```python
from build123d import *

# Parameters (mm, degrees)
BOSS_EXTRUDE1_DEPTH      = 1.5
SKETCH2_W                = 14
SKETCH2_H                = 32
BOSS_EXTRUDE2_DEPTH      = 16
BOSS_EXTRUDE3_DEPTH      = 3
BOSS_EXTRUDE3_DEPTH_BACK = 0.001
SKETCH3_W                = 15.664729633
SKETCH3_H                = 27
SKETCH3_R                = 1.75
SKETCH5_R                = 2.5
BOSS_EXTRUDE4_DEPTH      = 4
BOSS_EXTRUDE4_TAPER      = 15
CUT_EXTRUDE1_DEPTH       = 10
SKETCH7_W                = 71.065748979
SKETCH7_H                = 70.277880365
CUT_EXTRUDE2_DEPTH       = 30


with BuildPart() as part:
    # Sketch1 → Boss-Extrude1 (new body)
    with BuildSketch(Plane.YZ):
        Polygon((-13.5, 8), (-13.5, -8), (13.5, -8), (13.5, 8), (5, 8), (5, 58), (-5, 58), (-5, 8), align=None)
    extrude(amount=-BOSS_EXTRUDE1_DEPTH)



with BuildPart() as body_2:
    # Sketch2 → Boss-Extrude2 (new body)
    with BuildSketch(Plane.YZ):
        with Locations((0, -24)):
            Rectangle(SKETCH2_W, SKETCH2_H)
    extrude(amount=BOSS_EXTRUDE2_DEPTH)


with BuildPart() as part_1:
    add(part.part)

    add(body_2.part)  # Boss-Extrude3 merges body 2
    # Sketch3 → Boss-Extrude3 (add, two sides: drawn at the far end of the back side and taken through both)
    with BuildSketch(Plane.XY.offset(-8).offset(-BOSS_EXTRUDE3_DEPTH_BACK)):
        with Locations((6.299899253, 0)):
            Rectangle(SKETCH3_W, SKETCH3_H)
        with Locations((9.132264069, 9)):
            Circle(SKETCH3_R, mode=Mode.SUBTRACT)
        with Locations((9.132264069, -9)):
            Circle(SKETCH3_R, mode=Mode.SUBTRACT)
    extrude(amount=BOSS_EXTRUDE3_DEPTH + BOSS_EXTRUDE3_DEPTH_BACK)

    # Sketch5 → Boss-Extrude4 (add)
    with BuildSketch(Plane(origin=(0, 0, -40), x_dir=(1, 0, 0), z_dir=(0, 0, -1))):
        with Locations((9, 0)):
            Circle(SKETCH5_R)
    extrude(amount=BOSS_EXTRUDE4_DEPTH, taper=BOSS_EXTRUDE4_TAPER)

    # Sketch6 → Cut-Extrude1 (cut)
    with BuildSketch(Plane.YZ):
        with BuildLine():
            Line((0.555279177, 48), (0.555279177, 18))
            ThreePointArc((0.555279177, 18), (-1.194720823, 16.25), (-2.944720823, 18))
            Line((-2.944720823, 18), (-2.944720823, 48))
            ThreePointArc((-2.944720823, 48), (-1.194720823, 49.75), (0.555279177, 48))
        make_face()
    extrude(amount=-CUT_EXTRUDE1_DEPTH, mode=Mode.SUBTRACT)

    # Sketch7 → Cut-Extrude2 (cut)
    with BuildSketch(Plane.YZ.offset(14.132264069)):
        with Locations((0.078786861, 30.138940183)):
            Rectangle(SKETCH7_W, SKETCH7_H)
    extrude(amount=-CUT_EXTRUDE2_DEPTH, mode=Mode.SUBTRACT)


solid = part_1.part
```
Input: part model. Units: mm. Frame: model coordinates. A direction names the side the tool comes from. Give positions to 0.01 mm unless a question says otherwise; leave off trailing zeros. Loops run counter-clockwise (first coordinate to the right, second up) from the corner with the lowest first, then second, coordinate; pieces in that order, holes last.
1) Line query: L1, parallel to Z at x = 3.5, y = 9.25; L2, parallel to Y at x = 14, z = -23.5; L3, parallel to X at y = 0.5, z = -15.5. Output: solid intervals per line, ascending.
A:
L1: z = -8 to -5
L2: y = -7 to 7
L3: x = 0 to 16
2) Section query B-B on x = 2.5. Return the cut outline in (y, z).
A:
outline: (-13.5, -8) - (-7, -8) - (-7, -40) - (7, -40) - (7, -8) - (13.5, -8) - (13.5, -5) - (-13.5, -5) - close
3) Section query D-D on z = -34.5. Return the cut outline in (x, y), and give its area (3 significant figures).
A:
outline: (0, -7) - (16, -7) - (16, 7) - (0, 7) - close
area: 224 mm2
4) Section query A-A on y = 9. Return the cut outline in (x, z).
A:
outline: (-1.53, -8) - (7.38, -8) - (7.38, -5) - (-1.53, -5) - close; (10.88, -8) - (14.13, -8) - (14.13, -5) - (10.88, -5) - close
5) Mould query, pull axis X, two halves, no side actions, for faces 5 (the flat face through (0, 0, -24)), 6 (the cylindrical face through (8.904, 10.735, -6.522)), 7 (the flat face through (6, 0, -40)). Classes: released by +X, released by -X, zero draft, split by the parting line, or undercut.
A:
face 5: released by -X
face 6: undercut
face 7: zero draft
6) Section query C-C on x = 9. Return the cut outline in (y, z) (3 decimals).
A:
outline: (-13.5, -8.001) - (-10.745, -8.001) - (-10.745, -5) - (-13.5, -5) - close; (-7.255, -8.001) - (-7, -8.001) - (-7, -40) - (-2.5, -40) - (-1.428, -44) - (1.428, -44) - (2.5, -40) - (7, -40) - (7, -8.001) - (7.255, -8.001) - (7.255, -5) - (-7.255, -5) - close; (10.745, -8.001) - (13.5, -8.001) - (13.5, -5) - (10.745, -5) - close
7) Contact query for flat-ended pins moving along their axis: pin 1 (0.9 mm diameter, centred on x = 15, y = -0.5, fed in from +Z); pin 2 (5 mm diameter, centred on x = 8, z = -29.5, fed in from -Y); pin 3 (6 mm diameter, centred on x = 8, z = -28.5, fed in from +Y). Output: stop coordinate, or through.
A:
pin 1: stops at z = -8
pin 2: stops at y = -7
pin 3: stops at y = 7
8) Reachability of faces 1 (the flat face through (14.132, 0, -7)), 2 (the flat face through (-1, 0, -8.001)), 3 (the flat face through (8, -7, -24)), 4 (the flat face through (8, 7, -24)) from +Z, -Z, +X, -X, +Y, -Y: full face, straight path, thin tool, end or side. Return the list, or none.
A:
face 1: +Z, +X, +Y, -Y
face 2: -Z, -X
face 3: -Z, +X, -X, -Y
face 4: -Z, +X, -X, +Y
